Geometry: final body of the model. Coordinates: model frame, mm. Face numbers are marked on the shaded views. A direction names the side the tool comes from. Give positions to 0.01 mm unless a question says otherwise; leave off trailing zeros. Loops run counter-clockwise (first coordinate to the right, second up) from the corner with the lowest first, then second, coordinate; pieces in that order, holes last. Notation, with made-up numbers: (43.25, 76.5) -> (79.25, 76.5) arc R20 ccw to (79.25, 81.5) -> close; hole circle Ø8 at (73, -21.75). An arc over 180 degrees is marked (long way). Answer in a Markdown table with one row per item. Add a question column.
1) Section query B-B (x = -17). Return the cut outline in (y, z), plus the area to 3 significant figures.
2) Section query A-A (y = -8). Return the cut outline in (x, z), plus the area to 3 significant figures.
3) Draft query along X for the marked faces 1, 2 and 3. Return one class per face: +X half, -X half, draft (parallel to the pull), parting line (faces both ways), or undercut.
4) Access query for the marked faces 4, 5, 6 and 7. Directions: +Z, -Z, +X, -X, +Y, -Y. A direction counts if a zero-diameter tool reaches every point of the face in a straight line with its end or side. Return the directions, or none.
5) Section query D-D (x = -25). Return the cut outline in (y, z), plus the area to 3 significant figures.
6) Line query: line 1 (Y direction, x = -25, z = 16); line 2 (Y direction, x = -22, z = -14); line 3 (X direction, y = -6, z = 8). Output: solid intervals per line, ascending. Write a range as from..to.
7) First-contact query: P1, Ø8.5, axis at y = -12, z = 4.5, coming from the -X side; P2, Ø11, axis at x = -17.5, z = -17, coming from the +Y side; P3, Ø12, axis at y = -0.5, z = 2, coming from the +X side. Flat tips, straight axial feed; report the tip coordinate or a pass-through.
```python
from build123d import *

# Parameters (mm, degrees)
SKETCH2_R            = 2.98
BOSS_EXTRUDE1_DEPTH  = 20
FILLET1_R            = 6
FILLET2_R            = 2
FILLET4_R            = 5
SKETCH3_W            = 23.5
SKETCH3_H            = 9
SKETCH3_R            = 2.5
BOSS_EXTRUDE2_DEPTH  = 10
FILLET3_R            = 3
FILLET3_OF_MIRROR1_R = 3


with BuildPart() as part:
    # Sketch2 → Boss-Extrude1 (new, symmetric)
    with BuildSketch(Plane.XY):
        with BuildLine():
            Line((-6, 6), (6, 6))
            Line((6, 6), (6, -23.237900077))
            ThreePointArc((6, -23.237900077), (11.905106784, -20.839108245), (16.970562748, -16.970562748))
            Line((16.970562748, -16.970562748), (22.627416998, -22.627416998))
            ThreePointArc((22.627416998, -22.627416998), (18.117975616, -26.376864096), (13, -29.240383034))
            Line((13, -29.240383034), (-6, -18.27072792))
            Line((-6, -18.27072792), (-6, 6))
        make_face()
        Circle(SKETCH2_R, mode=Mode.SUBTRACT)
    extrude(amount=BOSS_EXTRUDE1_DEPTH, both=True)

    # Fillet1
    fillet1_edges = [part.edges().sort_by_distance(p)[0] for p in [
        (6, 6, 0),
        (-6, 6, 0),
    ]]
    fillet(fillet1_edges, radius=FILLET1_R - 0.0001)  # a hair under: the kernel refuses the full size

    # Fillet2
    fillet2_edges = [part.edges().sort_by_distance(p)[0] for p in [
        (16.970562748, -16.970562748, 0),
        (22.627416998, -22.627416998, 0),
        (13, -29.240383034, 0),
        (-6, -18.27072792, 0),
    ]]
    fillet(fillet2_edges, radius=FILLET2_R)

    # Fillet4
    fillet4_edges = [part.edges().sort_by_distance(p)[0] for p in [
        (6, -23.237900077, 0),
    ]]
    fillet(fillet4_edges, radius=FILLET4_R)

    # Sketch3 → Boss-Extrude2 (add)
    with BuildSketch(Plane.XY.offset(20)):
        with Locations((-17.75, -8)):
            Rectangle(SKETCH3_W, SKETCH3_H)
        with Locations((-25, -8)):
            Circle(SKETCH3_R, mode=Mode.SUBTRACT)
    boss_extrude2 = extrude(amount=-BOSS_EXTRUDE2_DEPTH)

    # Fillet3
    fillet3_edges = [part.edges().sort_by_distance(p)[0] for p in [
        (-6, -3.5, 15),
        (-6, -12.5, 15),
        (-29.5, -12.5, 15),
        (-29.5, -3.5, 15),
    ]]
    fillet(fillet3_edges, radius=FILLET3_R)

    # Mirror1: Boss-Extrude2 across plane
    add(boss_extrude2.mirror(Plane.XY))

    # Fillet3 of Mirror1
    fillet3_of_mirror1_edges = [part.edges().sort_by_distance(p)[0] for p in [
        (-6, -3.5, -15),
        (-6, -12.5, -15),
        (-29.5, -12.5, -15),
        (-29.5, -3.5, -15),
    ]]
    fillet(fillet3_of_mirror1_edges, radius=FILLET3_OF_MIRROR1_R)


solid = part.part
```
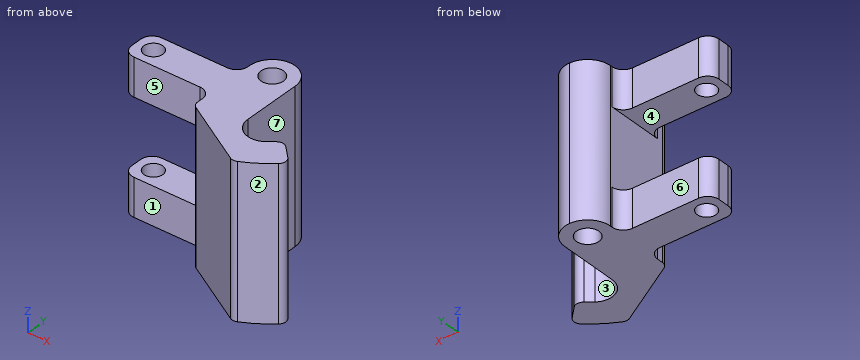
Evaluation:
| question | item | result |
|---|---|---|
| 1 | outline | (-12.5, -20) -> (-3.5, -20) -> (-3.5, -10) -> (-12.5, -10) -> close; (-12.5, 10) -> (-3.5, 10) -> (-3.5, 20) -> (-12.5, 20) -> close |
| 1 | area | 180 mm² |
| 2 | outline | (-29.5, -20) -> (-27.5, -20) -> (-27.5, -10) -> (-29.5, -10) -> close; (-29.5, 10) -> (-27.5, 10) -> (-27.5, 20) -> (-29.5, 20) -> close; (-22.5, -20) -> (6, -20) -> (6, 20) -> (-22.5, 20) -> (-22.5, 10) -> (-6, 10) -> (-6, -10) -> (-22.5, -10) -> close |
| 2 | area | 850 mm² |
| 3 | face 1 | draft |
| 3 | face 2 | +X half |
| 3 | face 3 | undercut |
| 4 | face 4 | -X, +Y, -Y |
| 4 | face 5 | +Z, -Z, -X, -Y |
| 4 | face 6 | +Z, -Z, -X, +Y |
| 4 | face 7 | +Z, -Z, +X, +Y |
| 5 | outline | (-12.5, -20) -> (-10.5, -20) -> (-10.5, -10) -> (-12.5, -10) -> close; (-12.5, 10) -> (-10.5, 10) -> (-10.5, 20) -> (-12.5, 20) -> close; (-5.5, -20) -> (-3.5, -20) -> (-3.5, -10) -> (-5.5, -10) -> close; (-5.5, 10) -> (-3.5, 10) -> (-3.5, 20) -> (-5.5, 20) -> close |
| 5 | area | 80.0 mm² |
| 6 | line 1 | -12.5..-10.5, -5.5..-3.5 |
| 6 | line 2 | -12.5..-3.5 |
| 6 | line 3 | -6..6 |
| 7 | P1 | x = -6 |
| 7 | P2 | y = -3.5 |
| 7 | P3 | x = 6 |
